Geometry: final body of the model. Coordinates: model frame, mm. Face numbers are marked on the shaded views. A direction names the side the tool comes from. Round coordinates to 2 decimals unless told otherwise and drop trailing zeros. Loops run counter-clockwise (first coordinate to the right, second up) from the corner with the lowest first, then second, coordinate; pieces in that order, holes last. Notation, with made-up numbers: (5.5, -36.5) -> (63.5, -36.5) arc R15 ccw to (63.5, -19.5) -> close; hole circle Ø6 at (58, 89.25). An arc over 180 degrees is marked (long way). Answer in a Markdown table with one row per item.
```python
from build123d import *

# Parameters (mm, degrees)
ESQUISSE1_R             = 150
ESQUISSE1_R_2           = 100
BOSS_EXTRU_1_DEPTH      = 50
ESQUISSE2_R             = 15
ENL_V_MAT_EXTRU_1_DEPTH = 40
ESQUISSE3_R             = 6
ENL_V_MAT_EXTRU_2_DEPTH = 10


with BuildPart() as part:
    # Esquisse1 → Boss.-Extru.1 (new body)
    with BuildSketch(Plane.XY):
        Circle(ESQUISSE1_R)
        Circle(ESQUISSE1_R_2, mode=Mode.SUBTRACT)
    extrude(amount=BOSS_EXTRU_1_DEPTH)

    # Esquisse2 → Enlèv. mat.-Extru.1 (cut)
    with BuildSketch(Plane.XY.offset(50)):
        with Locations((0, 125)):
            Circle(ESQUISSE2_R)
        with Locations((54.23546739, 112.621108488)):
            Circle(ESQUISSE2_R)
        with Locations((97.728935309, 77.936225232)):
            Circle(ESQUISSE2_R)
        with Locations((121.865989023, 27.815116745)):
            Circle(ESQUISSE2_R)
        with Locations((121.865989023, -27.815116745)):
            Circle(ESQUISSE2_R)
        with Locations((97.728935309, -77.936225232)):
            Circle(ESQUISSE2_R)
        with Locations((54.23546739, -112.621108488)):
            Circle(ESQUISSE2_R)
        with Locations((0, -125)):
            Circle(ESQUISSE2_R)
        with Locations((-54.23546739, -112.621108488)):
            Circle(ESQUISSE2_R)
        with Locations((-97.728935309, -77.936225232)):
            Circle(ESQUISSE2_R)
        with Locations((-121.865989023, -27.815116745)):
            Circle(ESQUISSE2_R)
        with Locations((-121.865989023, 27.815116745)):
            Circle(ESQUISSE2_R)
        with Locations((-97.728935309, 77.936225232)):
            Circle(ESQUISSE2_R)
        with Locations((-54.23546739, 112.621108488)):
            Circle(ESQUISSE2_R)
    extrude(amount=-ENL_V_MAT_EXTRU_1_DEPTH, mode=Mode.SUBTRACT)

    # Esquisse3 → Enlèv. mat.-Extru.2 (cut)
    with BuildSketch(Plane.XY.offset(10)):
        with Locations((0, 125)):
            Circle(ESQUISSE3_R)
        with Locations((54.23546739, 112.621108488)):
            Circle(ESQUISSE3_R)
        with Locations((97.728935309, 77.936225232)):
            Circle(ESQUISSE3_R)
        with Locations((121.865989023, 27.815116745)):
            Circle(ESQUISSE3_R)
        with Locations((121.865989023, -27.815116745)):
            Circle(ESQUISSE3_R)
        with Locations((97.728935309, -77.936225232)):
            Circle(ESQUISSE3_R)
        with Locations((54.23546739, -112.621108488)):
            Circle(ESQUISSE3_R)
        with Locations((0, -125)):
            Circle(ESQUISSE3_R)
        with Locations((-54.23546739, -112.621108488)):
            Circle(ESQUISSE3_R)
        with Locations((-97.728935309, -77.936225232)):
            Circle(ESQUISSE3_R)
        with Locations((-121.865989023, -27.815116745)):
            Circle(ESQUISSE3_R)
        with Locations((-121.865989023, 27.815116745)):
            Circle(ESQUISSE3_R)
        with Locations((-97.728935309, 77.936225232)):
            Circle(ESQUISSE3_R)
        with Locations((-54.23546739, 112.621108488)):
            Circle(ESQUISSE3_R)
    extrude(amount=-ENL_V_MAT_EXTRU_2_DEPTH, mode=Mode.SUBTRACT)


solid = part.part
```
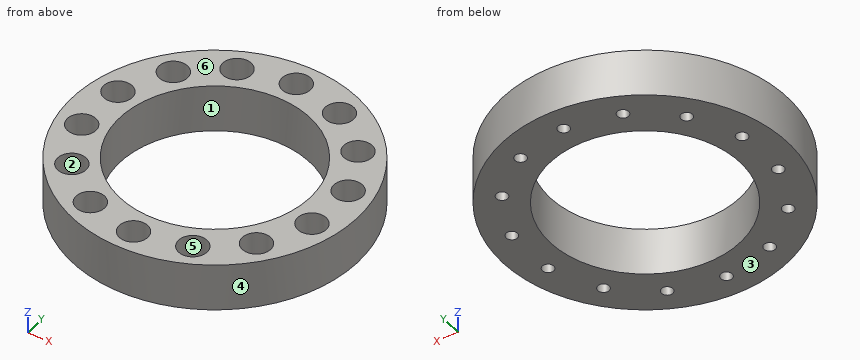
Item 1: Set-up query: the marked faces 5 and 6. Return all of +Z, -Z, +X, -X, +Y, -Y with unobstructed straight access to the full face (end or side cutting, diameter ignored); none if empty.
Ans:
| item | result |
|---|---|
| face 5 | +Z |
| face 6 | +Z, +X, -X, +Y, -Y |
Item 2: Section query D-D, the plane z = 32. State how many separate pieces and enclosed holes the cut face has, and give its area (3 significant figures).
Ans:
| item | result |
|---|---|
| separate pieces | 1 |
| enclosed holes | 15 |
| area | 29,400 mm2 |
Item 3: First-contact query: P1, Ø1.5, axis at y = 105, z = 26, coming from the -X side; P2, Ø1.5, axis at x = 23, z = 40.5, coming from the -Y side; P3, Ø24, axis at x = 97.73, y = -77.94, coming from the +Z side. Flat tips, straight axial feed; report the tip coordinate or a pass-through.
Ans:
| item | result |
|---|---|
| P1 | x = -107.85 |
| P2 | y = -148.34 |
| P3 | z = 10 |
Item 4: Mould query, pull axis Y, two halves, no side actions, for the marked faces 1, 2, 3 and 4. Classes: released by +Y, released by -Y, zero draft, split by the parting line, or undercut.
Ans:
| item | result |
|---|---|
| face 1 | undercut |
| face 2 | undercut |
| face 3 | zero draft |
| face 4 | split by the parting line |
Item 5: Section query A-A, the plane x = 0. Output: boundary loops of the cut face in (y, z).
Ans:
| item | result |
|---|---|
| outline | (-150, 0) -> (-131, 0) -> (-131, 10) -> (-140, 10) -> (-140, 50) -> (-150, 50) -> close; (-119, 0) -> (-100, 0) -> (-100, 50) -> (-110, 50) -> (-110, 10) -> (-119, 10) -> close; (100, 0) -> (119, 0) -> (119, 10) -> (110, 10) -> (110, 50) -> (100, 50) -> close; (131, 0) -> (150, 0) -> (150, 50) -> (140, 50) -> (140, 10) -> (131, 10) -> close |
Item 6: Section query B-B, the plane y = 0. Output: boundary loops of the cut face in (x, z), and give its area (3 significant figures).
Ans:
| item | result |
|---|---|
| outline | (-150, 0) -> (-100, 0) -> (-100, 50) -> (-150, 50) -> close; (100, 0) -> (150, 0) -> (150, 50) -> (100, 50) -> close |
| area | 5,000 mm2 |
Item 7: Ray query, L1, parallel to Y at x = 0, z = 7.5; L2, parallel to Y at x = -1, z = 12 (3 decimals); L3, parallel to Y at x = 121, z = 29. Return the intervals inside material, ascending.
Ans:
| item | result |
|---|---|
| L1 | -150 to -131, -119 to -100, 100 to 119, 131 to 150 |
| L2 | -149.997 to -139.967, -110.033 to -99.995, 99.995 to 110.033, 139.967 to 149.997 |
| L3 | -88.65 to -42.79, -12.84 to 12.84, 42.79 to 88.65 |
Item 8: Section query C-C, the plane x = -30.5. Output: boundary loops of the cut face in (y, z), and give its area (3 significant figures).
Ans:
| item | result |
|---|---|
| outline | (-146.87, 0) -> (-95.24, 0) -> (-95.24, 50) -> (-146.87, 50) -> close; (95.24, 0) -> (146.87, 0) -> (146.87, 50) -> (95.24, 50) -> close |
| area | 5,160 mm2 |
